Model file for the job. Use its own axes, mm. Round coordinates to 2 decimals unless told otherwise and drop trailing zeros. Order: outer loops, then holes, each group sorted by start corner. A loop starts at its lowest first (then second) coordinate and runs counter-clockwise, first axis right, second up. Notation, with made-up numbers: (4, 54) -> (42, 54) arc R22 cw to (42, 71) -> close; hole circle Ø10 at (86.5, 56). An arc over 180 degrees is marked (long way). Put each result on its own line as item: value. Start each with the question number.
Q1. Cut at C-C, the plane x = 53.5. List the corners of the cut face in (y, z), and give its area (3 significant figures).
Q2. Cut at A-A, the plane y = -23. List the corners of the cut face in (x, z).
Q3. Probe L1, parallel to Y at x = 89.5, z = 4.5; L2, parallel to X at y = 13, z = 5.75; L3, parallel to X at y = -24, z = 5.5. List the from-to ranges inside material, lowest first.
Q4. Cut at B-B, the plane y = 35.97. List the corners of the cut face in (x, z), and give its area (3 significant figures).
Q5. Flat gauge pins, fed straight in: P1, Ø2.5, axis at y = 12.5, z = 4, coming from the -X side; P2, Ø12, axis at x = 36, y = 55.5, coming from the -Z side; P3, Ø2.5, axis at y = 6.5, z = 2, coming from the +X side. Where does each tip first touch, or does it go through?
Q6. Cut at D-D, the plane z = 4.75. State how many separate pieces and enclosed holes the cut face has, and give its area (3 significant figures).
Autodesk Inventor part; units mm, degrees
ref_plane "YZ Plane" through (0, 0, 0) normal (1, 0, 0) x (0, 1, 0)
ref_plane "XZ Plane" through (0, 0, 0) normal (0, 1, 0) x (-1, 0, 0)
ref_plane "XY Plane" through (0, 0, 0) normal (0, 0, 1) x (1, 0, 0)
sketch "Sketch1" plane through (0, 0, 0) normal (0, 0, 1) x (1, 0, 0)
  circle A0 centre (-45.2437, 35.97) radius 3.175
  circle A1 centre (10.6363, 18.2563) radius 3.175
  line L0 (-71.7503, -2.6941) -> (-71.7503, 45.5566)
  line L1 (69.7183, -2.6941) -> (-71.7503, -2.6941)
  line L2 (69.7183, 45.5566) -> (69.7183, -2.6941)
  line L3 (-71.7503, 45.5566) -> (69.7183, 45.5566)
  line L4 (99.568, 75.4063) -> (99.568, -32.5437)
  line L5 (99.568, -32.5437) -> (-101.6, -32.5438)
  line L6 (-101.6, -32.5438) -> (-101.6, 75.4062)
  line L7 (-101.6, 75.4062) -> (99.568, 75.4063)
  line L8 (18.8383, 62.7063) -> (74.667, 62.7063)
  line L9 (74.667, 62.7063) -> (74.667, -26.1937)
  line L10 (74.667, -26.1937) -> (18.8383, -26.1937)
  line L11 (18.8383, -26.1937) -> (18.8383, 62.7063)
  line L12 (99.568, 21.4313) -> (-101.6, 21.4312) construction
  line L13 (8.6043, 3.175) -> (8.6043, 21.4313) construction
  point P0 (0, 0)
  dimension "d2" = 201.168
  dimension "d3" = 107.95
  dimension "d4" = 107.95
  dimension "d5" = 90
  dimension "d6" = 201.168
  dimension "d7" = 12.7
  dimension "d8" = 88.9
  dimension "d26" = 39.4363
  dimension "d27" = 56.3563
  dimension "d28" = 6.35
extrude "Extrusion1" add sketch "Sketch1" along normal blind 6.35 contours L0 L3 L11 L1 | L4 L5 L6 L7
sketch "Sketch2" plane through (0, 0, 0) normal (0, 0, -1) x (-1, 0, 0)
  line L0 (101.6, -32.5438) -> (101.6, 75.4062)
  line L1 (107.95, 65.692) -> (107.95, 61.9836)
  line L2 (107.95, 11.4304) -> (107.95, 7.722)
  line L3 (101.6, 7.722) -> (107.95, 7.722) construction
  line L4 (101.6, 11.4304) -> (107.95, 11.4304) construction
  line L5 (101.6, 61.9836) -> (107.95, 61.9836) construction
  line L6 (101.6, 65.4439) -> (107.95, 65.4439) construction
  line L7 (101.6, 7.722) -> (88.9, 7.722)
  line L8 (88.9, 7.722) -> (88.9, 11.4304)
  line L9 (88.9, 11.4304) -> (101.6, 11.4304)
  line L10 (101.6, 11.4304) -> (101.6, 7.722)
  line L11 (101.6, 61.9836) -> (88.9, 61.9836)
  line L12 (88.9, 61.9836) -> (88.9, 65.692)
  line L13 (88.9, 65.692) -> (101.6, 65.692)
  line L14 (101.6, 65.692) -> (101.6, 61.9836)
  line L15 (92.456, 5.6392) -> (95.25, 5.6392)
  line L16 (95.25, 5.6392) -> (95.25, 13.5132)
  line L17 (95.25, 13.5132) -> (92.456, 13.5132)
  line L18 (92.456, 13.5132) -> (92.456, 5.6392)
  line L19 (92.456, 59.9008) -> (95.25, 59.9008)
  line L20 (95.25, 59.9008) -> (95.25, 67.7748)
  line L21 (95.25, 67.7748) -> (92.456, 67.7748)
  line L22 (92.456, 67.7748) -> (92.456, 59.9008)
  point P0 (0, 0)
  dimension "d9" = 12.7
  dimension "d10" = 2.794
  dimension "d11" = 7.874
  dimension "d12" = 7.874
  dimension "d13" = 2.794
  dimension "d14" = 2.0828
  dimension "d16" = 2.0828
  dimension "d17" = 2.0828
  dimension "d18" = 6.35
  dimension "d19" = 6.35
extrude "Extrusion2" cut sketch "Sketch2" against normal through all
ref_plane "Work Plane1" through (-1.016, -32.5437, 0) normal (-1, 0, 0) x (0, 0, 1)
mirror "Mirror1" about plane through (-1.016, -32.5437, 0) normal (-1, 0, 0) of "Extrusion2"
sketch "Sketch3" plane through (-101.6, 11.4304, 0) normal (-1, 0, 0) x (0, 0, 1)
  line L0 (0, 0) -> (0, 50.5532)
  line L1 (6.35, 0) -> (6.35, 50.5532)
  line L2 (6.35, 12.5766) -> (0, 12.5766)
  line L3 (0, 37.9766) -> (6.35, 37.9766)
  point P0 (0, -11.4304)
extrude "Extrusion3" add sketch "Sketch3" along normal blind 6.35
ref_plane "Work Plane2" through (-1.016, 75.4062, 6.35) normal (1, 0, 0) x (0, 0, -1)
mirror "Mirror2" about plane through (-1.016, 75.4062, 6.35) normal (1, 0, 0) of "Extrusion3"
equation "\"d4\" = d3"
equation "\"d6\" = d2"
equation "\"d13\" = d10"
equation "\"d14\" = d16"
equation "\"d17\" = d14"
equation "\"d19\" = d18"
properties part number "projectorMountingBase_RB01" material "Steel, Wrought"
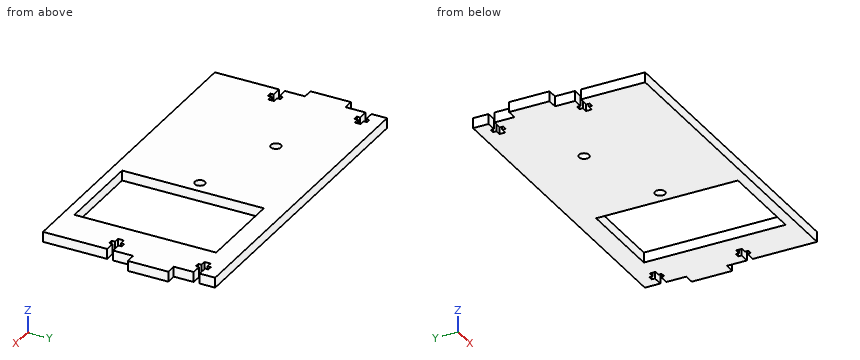
Ans:
1. outline: (-32.54, 0) -> (-26.19, 0) -> (-26.19, 6.35) -> (-32.54, 6.35) -> close; (62.71, 0) -> (75.41, 0) -> (75.41, 6.35) -> (62.71, 6.35) -> close
1. area: 121 mm^2
2. outline: (-101.6, 0) -> (18.84, 0) -> (18.84, 6.35) -> (-101.6, 6.35) -> close; (74.67, 0) -> (99.57, 0) -> (99.57, 6.35) -> (74.67, 6.35) -> close
3. L1: y = -32.54 to 7.72, 11.43 to 61.98, 65.69 to 75.41
3. L2: x = -101.6 to -95.25, -92.46 to 18.84, 74.67 to 90.42, 93.22 to 99.57
3. L3: x = -101.6 to 18.84, 74.67 to 99.57
4. outline: (-107.95, 0) -> (-48.42, 0) -> (-48.42, 6.35) -> (-107.95, 6.35) -> close; (-42.07, 0) -> (18.84, 0) -> (18.84, 6.35) -> (-42.07, 6.35) -> close; (74.67, 0) -> (105.92, 0) -> (105.92, 6.35) -> (74.67, 6.35) -> close
4. area: 963 mm^2
5. P1: stops at x = -101.6
5. P2: passes through
5. P3: stops at x = 99.57
6. separate pieces: 1
6. enclosed holes: 3
6. area: 16,800 mm^2
